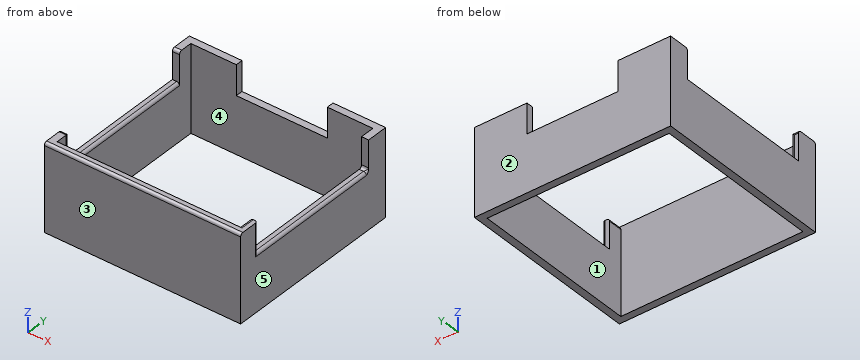
```python
from build123d import *

# Parameters (mm, degrees)
BOX002_W     = 200
BOX002_H     = 49
BOX002_DEPTH = 12
BOX003_W     = 32
BOX003_H     = 200
BOX003_DEPTH = 12
BOX_W        = 64
BOX_H        = 59
BOX_DEPTH    = 30.5
BOX001_W     = 69
BOX001_H     = 64
BOX001_DEPTH = 30.5
FILLET_R     = 1


with BuildPart() as cut_cube:
    # Box002 → Box002 (new body)
    with BuildSketch(Plane(origin=(-50, 7.5, 20), x_dir=(1, 0, 0), z_dir=(0, 0, 1))):
        with Locations((100, 24.5)):
            Rectangle(BOX002_W, BOX002_H)
    extrude(amount=BOX002_DEPTH)


with BuildPart() as cut_cube001:
    # Box003 → Box003 (new body)
    with BuildSketch(Plane(origin=(18.5, 7.5, 20), x_dir=(1, 0, 0), z_dir=(0, 0, 1))):
        with Locations((16, 100)):
            Rectangle(BOX003_W, BOX003_H)
    extrude(amount=BOX003_DEPTH)


with BuildPart() as fusion:
    # Box → Box (new body)
    with BuildSketch(Plane(origin=(2.5, 2.5, 0), x_dir=(1, 0, 0), z_dir=(0, 0, 1))):
        with Locations((32, 29.5)):
            Rectangle(BOX_W, BOX_H)
    extrude(amount=BOX_DEPTH)

    # Fusion: union cut cube, cut cube001
    add(cut_cube.part)
    add(cut_cube001.part)


with BuildPart() as fillet_body:
    # Box001 → Box001 (new body)
    with BuildSketch(Plane.XY):
        with Locations((34.5, 32)):
            Rectangle(BOX001_W, BOX001_H)
    extrude(amount=BOX001_DEPTH)

    # Cut: cut Fusion
    add(fusion.part, mode=Mode.SUBTRACT)

    # Fillet
    fillet_edges = [fillet_body.edges().sort_by_distance(p)[0] for p in [
        (1.25, 7.5, 30.5),
        (66.5, 5, 30.5),
        (34.5, 0, 30.5),
        (2.5, 7.5, 25.25),
        (2.5, 32, 20),
        (1.25, 56.5, 30.5),
        (69, 7.5, 25.25),
        (69, 32, 20),
        (67.75, 56.5, 20),
    ]]
    fillet(fillet_edges, radius=FILLET_R)


solid = fillet_body.part
```
Could you check a few things on this model? Use its own coordinates, in mm. Face numbers are marked on the shaded views. A direction names the side the tool comes from. Coordinates: 2 decimals unless noted, no trailing zeros. Write each loop counter-clockwise with the first axis right and the second up, starting at its lowest first coordinate (ties: lowest second). Pieces come first, ordered by that corner, then holes. Notation, with made-up numbers: (5.5, 48) - (51.5, 48) arc R12 ccw to (51.5, 56) - close; hole circle Ø10 at (27, -19). An arc over 180 degrees is marked (long way). Use a Markdown table: item, result.
Q1. I'm going to push flat-ended pins straight in: pin 1 Ø0.8 at (x, y) = (0.5, 25.5) entering from +Z; pin 2 Ø0.8 at (y, z) = (63, 25.5) entering from -X. Where does each tip first touch, or does it pass through?
Geometry check:
| item | result |
|---|---|
| pin 1 | stops at z = 20 |
| pin 2 | stops at x = 0 |
Q2. Which directions (+Z, -Z, +X, -X, +Y, -Y) give clear straight access to the entire face, cutting with the end or side of a thin tool? Please do the marked faces 1 and 2.
Geometry check:
| item | result |
|---|---|
| face 1 | +Z, -Z |
| face 2 | +Z, -Z, +X, -X, +Y |
Q3. Thinking about a two-plate mould opening in Y: for the marked faces 3, 4 and 5, which applies, +Y half, -Y half, draft (parallel to the pull), parting line (faces both ways), or undercut?
Geometry check:
| item | result |
|---|---|
| face 3 | -Y half |
| face 4 | undercut |
| face 5 | draft |
Q4. Imagine slicing it at C-C (z = 23.5). List the corners of the cut face in (x, y) for me, and give its area (3 significant figures).
Geometry check:
| item | result |
|---|---|
| outline | (0, 0) - (69, 0) - (69, 6.5) arc R1 ccw to (68, 7.5) - (66.5, 7.5) - (66.5, 2.5) - (2.5, 2.5) - (2.5, 6.5) arc R1 ccw to (1.5, 7.5) - (0, 7.5) - close; (0, 56.5) - (2.5, 56.5) - (2.5, 61.5) - (18.5, 61.5) - (18.5, 64) - (0, 64) - close; (50.5, 61.5) - (66.5, 61.5) - (66.5, 56.5) - (69, 56.5) - (69, 64) - (50.5, 64) - close |
| area | 315 mm2 |
Q5. Imagine slicing it at A-A (x = 45). List the corners of the cut face in (y, z) for me.
Geometry check:
| item | result |
|---|---|
| outline | (0, 0) - (2.5, 0) - (2.5, 30.5) - (1, 30.5) arc R1 ccw to (0, 29.5) - close; (61.5, 0) - (64, 0) - (64, 20) - (61.5, 20) - close |
Q6. Imagine slicing it at B-B (y = 31.5). List the corners of the cut face in (x, z) for me, and give its area (3 significant figures).
Geometry check:
| item | result |
|---|---|
| outline | (0, 0) - (2.5, 0) - (2.5, 19) arc R1 ccw to (1.5, 20) - (0, 20) - close; (66.5, 0) - (69, 0) - (69, 19) arc R1 ccw to (68, 20) - (66.5, 20) - close |
| area | 99.6 mm2 |
Q7. Imagine slicing it at D-D (z = 15). List the corners of the cut face in (x, y) for me, and give its area (3 significant figures).
Geometry check:
| item | result |
|---|---|
| outline | (0, 0) - (69, 0) - (69, 64) - (0, 64) - close; hole (2.5, 2.5) - (66.5, 2.5) - (66.5, 61.5) - (2.5, 61.5) - close |
| area | 640 mm2 |
Q8. Please list where these lines run through material, in increasing order: L1, parallel to X at y = 24, z = 17; L2, parallel to Y at x = 9.5, z = 20.5; L3, parallel to X at y = 7, z = 23.
Geometry check:
| item | result |
|---|---|
| L1 | x = 0 to 2.5, 66.5 to 69 |
| L2 | y = 0 to 2.5, 61.5 to 64 |
| L3 | x = 0 to 2.37, 66.5 to 68.87 |
